Build history of the part. All positions in model axes, mm. Face numbers are marked on the shaded views. A direction names the side the tool comes from. Coordinates: 2 decimals unless noted, no trailing zeros. Order: outer loops, then holes, each group sorted by start corner. A loop starts at its lowest first (then second) coordinate and runs counter-clockwise, first axis right, second up. Notation, with made-up numbers: M -23,-24.5 L 34,-24.5 A21 cw 34,8.5 Z; hole C 31,72 d6. An arc over 180 degrees is marked long. Write item = value, one per line. Start each with the question number.
Q1. Drill centre lines: probe 1 along Y at (x, z) = (3.15, -4); probe 2 along Z at (x, y) = (2.7, 0.25); probe 3 along Y at (x, z) = (3.15, -0.25). Where is each one in solid material? Low to high.
Q2. Band-saw the part on C-C on y = 6. Write the cut outline in (x, z), plus the area to 3 significant figures.
Q3. Pin check, flat tip, straight feed: P1, Ø1, axis at x = 0.5, y = -3, coming from the +Z side. Stop position of the tip, or through.
Q4. Band-saw the part on B-B on x = 2.45. Write the cut outline in (y, z), plus the area to 3 significant figures.
Q5. 3-axis set-ups, long thin cutter, end or side, ignore diameter. For the marked faces 1, 2, 3 and 4: which of +Z, -Z, +X, -X, +Y, -Y reach the whole face in a straight line?
Q6. Band-saw the part on D-D on y = -3. Write the cut outline in (x, z), plus the area to 3 significant figures.
Q7. Band-saw the part on A-A on z = 0. Write the cut outline in (x, y), plus the area to 4 significant figures.
Q8. Pull direction Z, two halves, no side cores. Call the marked faces 5, 6 and 7: released by +Z, released by -Z, zero draft, split by the parting line, or undercut.
Autodesk Inventor part; units mm, degrees
ref_plane "YZ Plane" through (0, 0, 0) normal (1, 0, 0) x (0, 1, 0)
ref_plane "XZ Plane" through (0, 0, 0) normal (0, 1, 0) x (-1, 0, 0)
ref_plane "XY Plane" through (0, 0, 0) normal (0, 0, 1) x (1, 0, 0)
sketch "Sketch1" plane through (0, 0, 0) normal (1, 0, 0) x (0, 1, 0)
  circle A0 centre (0, 0) radius 1.75
  circle A1 centre (0, 0) radius 5
  dimension "d0" = 3.5
  dimension "d1" = 10
extrude "Extrusion1" add sketch "Sketch1" along normal blind 3.5
sketch "Sketch2" plane through (3.5, 0, 0) normal (1, 0, 0) x (0, 0, -1)
  circle A0 centre (0, 0) radius 5 construction
  line L0 (0, 5) -> (0, 4.5) construction
  line L1 (0, 4.5) -> (1, 4.5) construction
  line L2 (1, 4.5) -> (-1, 4.5) construction
  line L3 (0, 4.5) -> (0, 7.5) construction
  arc A1 (0, 7.5) -> (-1, 4.5) centre (2.4623, 5.0126) ccw
  line L4 (0, 7.5) -> (2, 7.5)
  dimension "d4" = 0.5
  dimension "d5" = 1
  dimension "d6" = 2
  dimension "d7" = 3
  dimension "d8" = 3.5
  dimension "d9" = 2
sketch "Sketch3" plane through (3.5, 0, 0) normal (1, 0, 0) x (0, 0, -1)
  circle A0 centre (0, 0) radius 5 construction
  line L0 (-5, 0) -> (-4.5, 0) construction
  line L1 (-4.5, 0) -> (-4.5, 1.5) construction
  line L2 (-4.5, 1.5) -> (-4.5, 0) construction
  line L3 (-4.5, 0) -> (-4.5, -1.5) construction
  line L4 (-5, 0) -> (-7.5, 0) construction
  line L5 (-7.5, 0) -> (-4.5, -1.5)
  line L6 (-7.5, 0) -> (-7.5, 2)
  line L7 (-7.5, 2) -> (-4.9474, 0.7237)
  line L8 (-4.5, -1.5) -> (-4.5, 0.5)
  line L9 (-4.9474, 0.7237) -> (-4.5, 0.5)
  dimension "d10" = 0.5
  dimension "d11" = 1.5
  dimension "d12" = 1.5
  dimension "d13" = 1.5
  dimension "d14" = 2.5
  dimension "d15" = 2
extrude "Extrusion2" add sketch "Sketch3" against normal blind 3.5
pattern_circular "Circular Pattern1" count 6 over 360 about axis through (0, 0, 0) along (1, 0, 0) of "Extrusion2"
properties part number "mtv_gear6_1-16"
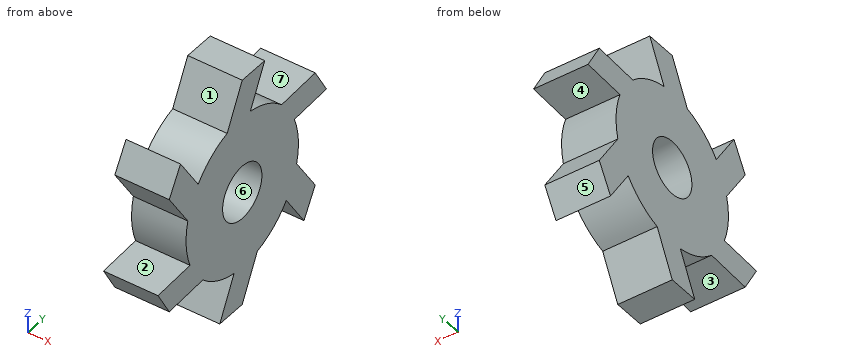
Recorded:
q1.probe_1 = -3 to 3, 4.52 to 6.35
q1.probe_2 = -7 to -1.73, 1.73 to 7.5
q1.probe_3 = -4.99 to -1.73, 1.73 to 4.99
q2.outline = M 0,-4.61 L 3.5,-4.61 L 3.5,-3 L 0,-3 Z; M 0,1.93 L 3.5,1.93 L 3.5,3.72 L 0,3.72 Z
q2.area = 11.9 mm2
q3.P1 = 4.33
q4.outline = M -7.5,-2.02 L -6.5,-3.75 L -3.5,-3.57 A5 ccw -0.72,-4.95 L -2,-7.5 L 0,-7.5 L 1.34,-4.82 A5 ccw 3.92,-3.1 L 5.5,-5.48 L 6.5,-3.75 L 4.84,-1.25 A5 ccw 4.65,1.85 L 7.5,2.02 L 6.5,3.75 L 3.5,3.57 A5 ccw 0.72,4.95 L 2,7.5 L 0,7.5 L -1.34,4.82 A5 ccw -3.92,3.1 L -5.5,5.48 L -6.5,3.75 L -4.84,1.25 A5 ccw -4.65,-1.85 Z; hole C 0,0 d3.5
q4.area = 99.4 mm2
q5.face_1 = +Z, +X, -X
q5.face_2 = +X, -X, -Y
q5.face_3 = -Z, +X, -X
q5.face_4 = +X, -X, +Y
q6.outline = M 0,-4 L 3.5,-4 L 3.5,4 L 0,4 Z
q6.area = 28.0 mm2
q7.outline = M 0,-5 L 3.5,-5 L 3.5,-1.75 L 0,-1.75 Z; M 0,1.75 L 3.5,1.75 L 3.5,5 L 0,5 Z
q7.area = 22.75 mm2
q8.face_5 = released by -Z
q8.face_6 = undercut
q8.face_7 = released by +Z
